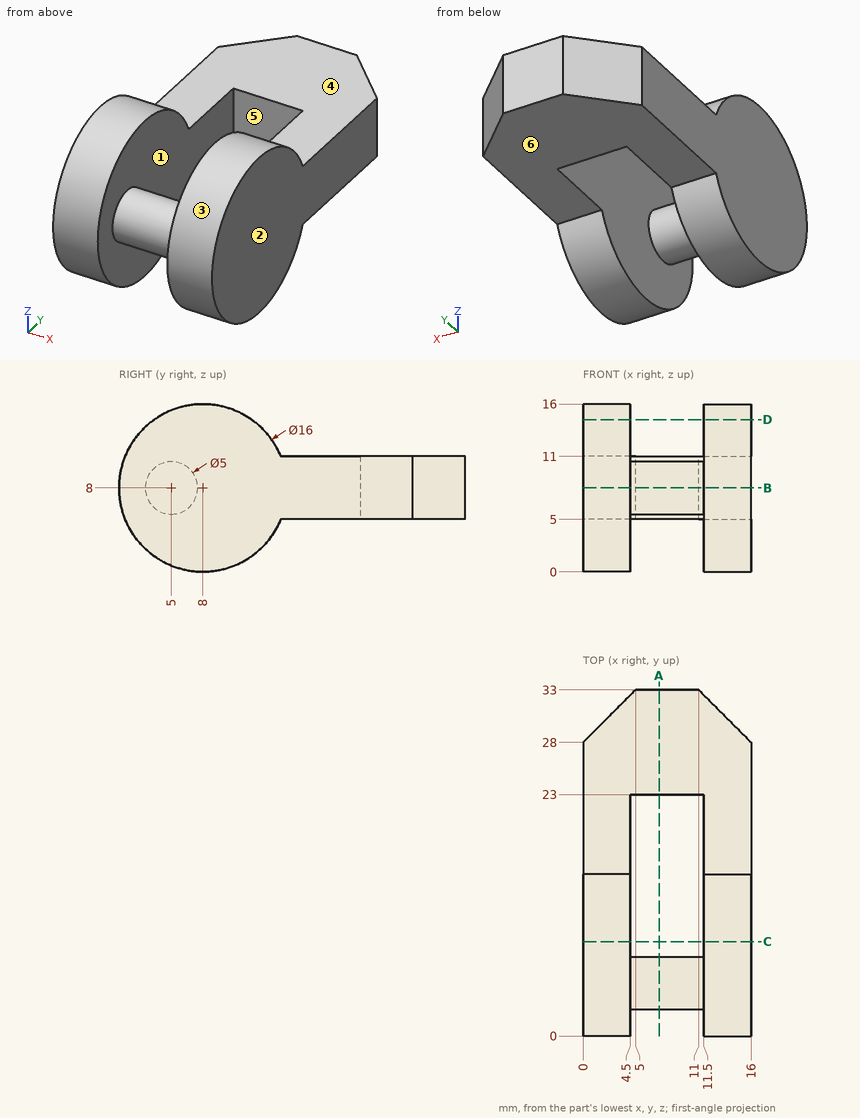
Job drawing, mm, ordinate dimensions from the low corner. One solid piece. A direction names the side the tool comes from. Coordinates: 2 decimals unless noted, no trailing zeros. Order: outer loops, then holes, each group sorted by start corner. A loop starts at its lowest first (then second) coordinate and runs counter-clockwise, first axis right, second up. Notation, with made-up numbers: (-1, 33.25) -> (19, 33.25) arc R21 cw to (19, 48.25) -> close; hole circle Ø1 at (-13, 26). An arc over 180 degrees is marked (long way). Put each result on its own line as item: value. Start each with the question number.
(1) Band-saw the part on C-C (y = 9). Give the cut face in (x, z), then the cut area to 3 significant figures.
(2) Band-saw the part on D-D (z = 14.5). Give the cut face in (x, y), then the cut area to 3 significant figures.
(3) Which spindle directions (+Z, -Z, +X, -X, +Y, -Y) get a long thin tool onto all of the face, cutting with end or side? Do the marked faces 4, 5 and 6. Say none if no direction does.
(4) Band-saw the part on B-B (z = 8). Give the cut face in (x, y).
(5) Pin check, flat tips, straight feed: pin 1 Ø2 at (x, z) = (3, 10) entering from -Y; pin 2 Ø4 at (x, y) = (4, 27) entering from +Z; pin 3 Ø4 at (x, y) = (2, 27.5) entering from -Z. Stop position of each tip, or through.
(6) Mould opens along X. For the marked faces 1, 2 and 3 say: pulls with the +X half, pulls with the -X half, needs draft (parallel to the pull), parting line crosses it, or undercut.
(7) Probe line 1 along X through (y, z) = (11, 8); line 2 along Y through (x, z) = (5, 8); line 3 along Z through (x, y) = (3.75, 25). List the from-to ranges inside material, lowest first. Write a range as [from, to].
(8) Band-saw the part on A-A (x = 7.25). Give the cut face in (y, z).
Determined:
1. outline: (0, 0.06) -> (4.5, 0.06) -> (4.5, 15.94) -> (0, 15.94) -> close; (11.5, 0.06) -> (16, 0.06) -> (16, 15.94) -> (11.5, 15.94) -> close
1. area: 143 mm²
2. outline: (0, 3.34) -> (4.5, 3.34) -> (4.5, 12.66) -> (0, 12.66) -> close; (11.5, 3.34) -> (16, 3.34) -> (16, 12.66) -> (11.5, 12.66) -> close
2. area: 83.9 mm²
3. face 4: +Z, +X, -X, +Y
3. face 5: +Z, -Z
3. face 6: -Z, +X, -X, +Y
4. outline: (0, 0) -> (4.5, 0) -> (4.5, 2.5) -> (11.5, 2.5) -> (11.5, 0) -> (16, 0) -> (16, 28) -> (11, 33) -> (5, 33) -> (0, 28) -> close; hole (4.5, 7.5) -> (11.5, 7.5) -> (11.5, 23) -> (4.5, 23) -> close
5. pin 1: stops at y = 0.06
5. pin 2: stops at z = 11
5. pin 3: stops at z = 5
6. face 1: undercut
6. face 2: pulls with the +X half
6. face 3: needs draft
7. line 1: x = [0, 4.5], [11.5, 16]
7. line 2: y = [2.5, 7.5], [23, 33]
7. line 3: z = [5, 11]
8. outline: circle Ø5 at (5, 8); (23, 5) -> (33, 5) -> (33, 11) -> (23, 11) -> close
